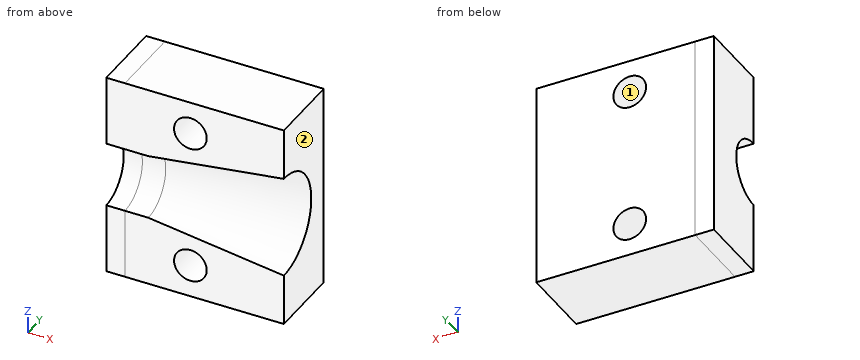
```python
from build123d import *

# Parameters (mm, degrees)
SKETCH_1_W          = 17
SKETCH_1_H          = 22
SKETCH_1_R          = 1.75
EXTRUDE_1_DEPTH     = 4
SKETCH_2_R          = 3.5
CUT_EXTRUDE_1_DEPTH = 2.5
SKETCH_4_R          = 5.5
SKETCH_3_R          = 3.5
EXTRUDE_2_DEPTH     = 2


with BuildPart() as part:
    # 草圖1 → 填料-伸長1 (new body, symmetric)
    with BuildSketch(Plane(origin=(0, 0, 0), x_dir=(1, 0, 0), z_dir=(0, 1, 0))):
        Rectangle(SKETCH_1_W, SKETCH_1_H)
        with Locations((-1.5, 7.5)):
            Circle(SKETCH_1_R, mode=Mode.SUBTRACT)
        with Locations((-1.5, -7.5)):
            Circle(SKETCH_1_R, mode=Mode.SUBTRACT)
    extrude(amount=EXTRUDE_1_DEPTH, both=True)

    # 草圖2 → 除料-伸長1 (cut)
    with BuildSketch(Plane.ZY.offset(8.5)):
        with Locations((0, -4)):
            Circle(SKETCH_2_R)
    extrude(amount=-CUT_EXTRUDE_1_DEPTH, mode=Mode.SUBTRACT)

    # 草圖4 → 除料-疊層拉伸1 section 0
    with BuildSketch(Plane(origin=(8.5, 0, 0), x_dir=(0, 0, -1), z_dir=(1, 0, 0))):
        with Locations((0, -4)):
            Circle(SKETCH_4_R)
    # 草圖3 → 除料-疊層拉伸1 section 1
    with BuildSketch(Plane.ZY.offset(6)):
        with Locations((0, -4)):
            Circle(SKETCH_3_R)
    loft(mode=Mode.SUBTRACT)

    # 草圖5 → 填料-伸長2 (add)
    with BuildSketch(Plane.ZY.offset(8.5)):
        with BuildLine():
            Line((3.5, -4), (11, -4))
            Line((11, -4), (11, 4))
            Line((11, 4), (-11, 4))
            Line((-11, 4), (-11, -4))
            Line((-11, -4), (-3.5, -4))
            ThreePointArc((-3.5, -4), (0, -0.5), (3.5, -4))
        make_face()
    extrude(amount=EXTRUDE_2_DEPTH)


solid = part.part
```
The listing builds one solid part. Answer for the finished solid, in the listing's coordinates (mm). Face numbers are marked on the shaded views. Round coordinates to 2 decimals unless told otherwise and drop trailing zeros. Order: outer loops, then holes, each group sorted by start corner. A loop starts at its lowest first (then second) coordinate and runs counter-clockwise, first axis right, second up. Notation, with made-up numbers: (1, 65.25) -> (47, 65.25) arc R36 ccw to (47, 101.25) -> close; hole circle Ø3 at (-25.75, 36). An arc over 180 degrees is marked (long way). Answer as CSV lines item,"result".
Q1. A cutting plane is placed at D-D on z = 0. Determine the outline of the cut face in (x, y), plus the area to 3 significant figures.
Computed values:
outline,"(-10.5, -0.5) -> (-6, -0.5) -> (8.5, 1.5) -> (8.5, 4) -> (-10.5, 4) -> close"
area,"71.0 mm^2"
Q2. Consider line 1 (Z direction, x = -3, y = 1.5); line 2 (X direction, y = 0, z = 7.5); line 3 (Z direction, x = -1.5, y = -0.75). Determine where each line is inside the solid, lowest interval first. Write a range as from..to.
Computed values:
line 1,"z = -11..-8.4, -6.6..6.6, 8.4..11"
line 2,"x = -10.5..-3.25, 0.25..8.5"
line 3,"z = -11..-9.25, -5.75..-2.53, 2.53..5.75, 9.25..11"
Q3. A cutting plane is placed at B-B on x = -1.5. Determine the outline of the cut face in (y, z).
Computed values:
outline,"(-4, -11) -> (4, -11) -> (4, -9.25) -> (-4, -9.25) -> close; (-4, -5.75) -> (4, -5.75) -> (4, 5.75) -> (-4, 5.75) -> (-4, 4.12) arc R4.12 cw to (-4, -4.12) -> close; (-4, 9.25) -> (4, 9.25) -> (4, 11) -> (-4, 11) -> close"
Q4. A cutting plane is placed at C-C on y = -2. Give the number of separate pieces and of enclosed holes in the cut face, plus the area to 3 significant figures.
Computed values:
separate pieces,"2"
enclosed holes,"2"
area,"256 mm^2"
Q5. For a pull along Z with two mould halves and no side action, classify the marked faces 1 and 2 as +Z half, -Z half, draft (parallel to the pull), parting line (faces both ways), or undercut.
Computed values:
face 1,"undercut"
face 2,"draft"
Q6. A cutting plane is placed at A-A on z = 7.5. Determine the outline of the cut face in (x, y), plus the area to 3 significant figures.
Computed values:
outline,"(-10.5, -4) -> (-3.25, -4) -> (-3.25, 4) -> (-10.5, 4) -> close; (0.25, -4) -> (8.5, -4) -> (8.5, 4) -> (0.25, 4) -> close"
area,"124 mm^2"
